Source: CAD feature listing. Evaluate the final solid. Frame: model axes, mm. A direction names the side the tool comes from. Round coordinates to 2 decimals unless told otherwise and drop trailing zeros. Write each loop counter-clockwise with the first axis right and the second up, starting at its lowest first coordinate (ties: lowest second). Pieces come first, ordered by that corner, then holes. Notation, with made-up numbers: M -5.5,-15.75 L -1.5,-15.75 A11 cw -1.5,-8.75 Z; hole C -19,-1.5 d9. An arc over 180 degrees is marked long. Answer in a Markdown table with one row per item. Add a question column.
Item 1: Contact query for flat-ended pins moving along their axis: pin 1 (0.5 mm diameter, centred on x = 37, y = 32.5, fed in from -Z); pin 2 (0.5 mm diameter, centred on x = 52.5, z = 2, fed in from +Y); pin 3 (2.5 mm diameter, centred on x = 48, y = 10, fed in from +Z); pin 4 (1.7 mm diameter, centred on x = 55, y = 30.5, fed in from -Z). Output: stop coordinate, or through.
Item 2: Cut plane A-A on x = 48. Return loops of the section in (y, z), and give its area (3 significant figures).
Item 3: Mould query, pull axis X, two halves, no side actions, for faces 6 (the face through (61.802, 0.713, 2.958)), 7 (the face through (0, 17, 4)), 8 (the face through (39, 17, 8)). Classes: released by +X, released by -X, zero draft, split by the parting line, or undercut.
Item 4: Cut plane D-D on x = 66.5. Return loops of the section in (y, z).
Item 5: Material intervals for probe 1 along X at (y, z) = (3, 2.25); probe 2 along Y at (x, z) = (73, 5.25); probe 3 along Y at (x, z) = (23, 7), sorted ascending.
Item 6: Cut plane C-C on x = 57. Return loops of the section in (y, z).
Item 7: Cut plane B-B on y = 25. Return loops of the section in (x, z).
Item 8: Set-up query: faces 1 (the face through (25, 6, 6)), 2 (the face through (52.35, 10.06, 2.22)), 3 (the face through (40, 33.2, 3)), 4 (the face through (76.74, 6.45, 3.94)), 5 (the face through (41, 33, 2.5)). Return all of +Z, -Z, +X, -X, +Y, -Y with unobstructed straight access to the full face (end or side cutting, diameter ignored); none if empty.
from build123d import *

# Parameters (mm, degrees)
SKETCH_2_W           = 80
SKETCH_2_H           = 34
SKETCH_2_R           = 4.05
EXTRUDE_1_DEPTH      = 8
SKETCH_3_R           = 2.55
CUT_EXTRUDE_1_DEPTH  = 88.292611371
CUT_EXTRUDE_2_DEPTH  = 88.292611371
SKETCH_5_R           = 1.55
CUT_EXTRUDE_3_DEPTH  = 88.292611371
CUT_EXTRUDE_4_DEPTH  = 6
CUT_EXTRUDE_5_DEPTH  = 4.5
SKETCH_20_R          = 5.5
CUT_EXTRUDE_12_DEPTH = 4.5
SKETCH_11_R          = 1.55
CUT_EXTRUDE_7_DEPTH  = 88.292611371
CUT_EXTRUDE_11_DEPTH = 2


with BuildPart() as part:
    # 草图2 → 凸台-拉伸1 (new body)
    with BuildSketch(Plane.XY):
        with Locations((40, 17)):
            Rectangle(SKETCH_2_W, SKETCH_2_H)
        with Locations((7, 8)):
            Circle(SKETCH_2_R, mode=Mode.SUBTRACT)
        with Locations((40, 10)):
            Circle(SKETCH_2_R, mode=Mode.SUBTRACT)
        with Locations((73, 8)):
            Circle(SKETCH_2_R, mode=Mode.SUBTRACT)
    extrude(amount=EXTRUDE_1_DEPTH)

    # 草图3 → 切除-拉伸1 (cut, through all)
    with BuildSketch(Plane.XY.offset(8)):
        with Locations((23, 8)):
            Circle(SKETCH_3_R)
        with Locations((57, 8)):
            Circle(SKETCH_3_R)
    extrude(amount=-CUT_EXTRUDE_1_DEPTH, mode=Mode.SUBTRACT)

    # 草图4 → 切除-拉伸2 (cut, through all)
    with BuildSketch(Plane(origin=(80, 0, 0), x_dir=(0, 0, -1), z_dir=(1, 0, 0))):
        Polygon((-1.5, 32.2), (-2.5, 32.2), (-2.5, 34), (0, 34), (0, 28.8), (-1.5, 28.8), align=None)
    extrude(amount=-CUT_EXTRUDE_2_DEPTH, mode=Mode.SUBTRACT)

    # 草图5 → 切除-拉伸3 (cut, through all)
    with BuildSketch(Plane.XY.offset(8)):
        with Locations((48, 10)):
            Circle(SKETCH_5_R)
        with Locations((32, 10)):
            Circle(SKETCH_5_R)
    extrude(amount=-CUT_EXTRUDE_3_DEPTH, mode=Mode.SUBTRACT)

    # 草图7 → 切除-拉伸4 (cut)
    with BuildSketch(Plane(origin=(0, 0, 0), x_dir=(-1, 0, 0), z_dir=(0, 0, -1))):
        with BuildLine():
            Line((-27.05, 10), (-27.05, 2.5))
            ThreePointArc((-27.05, 2.5), (-27.782233047, 0.732233047), (-29.55, 0))
            Line((-29.55, 0), (-16.45, 0))
            ThreePointArc((-16.45, 0), (-18.217766953, 0.732233047), (-18.95, 2.5))
            Line((-18.95, 2.5), (-18.95, 10))
            ThreePointArc((-18.95, 10), (-23, 14.05), (-27.05, 10))
        make_face()
        with BuildLine():
            Line((-61.05, 2.5), (-61.05, 10))
            ThreePointArc((-61.05, 10), (-57, 14.05), (-52.95, 10))
            Line((-52.95, 10), (-52.95, 2.5))
            ThreePointArc((-52.95, 2.5), (-52.217766953, 0.732233047), (-50.45, 0))
            Line((-50.45, 0), (-63.55, 0))
            ThreePointArc((-63.55, 0), (-61.782233047, 0.732233047), (-61.05, 2.5))
        make_face()
    extrude(amount=-CUT_EXTRUDE_4_DEPTH, mode=Mode.SUBTRACT)

    # 草图8 → 切除-拉伸5 (cut)
    with BuildSketch(Plane(origin=(0, 0, 0), x_dir=(-1, 0, 0), z_dir=(0, 0, -1))):
        with BuildLine():
            Line((-30.5, 12.85), (-49.5, 12.85))
            ThreePointArc((-49.5, 12.85), (-52.35, 10), (-49.5, 7.15))
            Line((-49.5, 7.15), (-30.5, 7.15))
            ThreePointArc((-30.5, 7.15), (-27.65, 10), (-30.5, 12.85))
        make_face()
    extrude(amount=-CUT_EXTRUDE_5_DEPTH, mode=Mode.SUBTRACT)

    # 草图20 → 切除-拉伸12 (cut)
    with BuildSketch(Plane(origin=(0, 0, 0), x_dir=(-1, 0, 0), z_dir=(0, 0, -1))):
        with Locations((-40, 10)):
            Circle(SKETCH_20_R)
    extrude(amount=-CUT_EXTRUDE_12_DEPTH, mode=Mode.SUBTRACT)

    # 草图11 → 切除-拉伸7 (cut, through all)
    with BuildSketch(Plane(origin=(0, 0, 0), x_dir=(-1, 0, 0), z_dir=(0, 0, -1))):
        with Locations((-60, 25)):
            Circle(SKETCH_11_R)
        with Locations((-20, 25)):
            Circle(SKETCH_11_R)
    extrude(amount=-CUT_EXTRUDE_7_DEPTH, mode=Mode.SUBTRACT)

    # 草图19 → 切除-拉伸11 (cut)
    with BuildSketch(Plane(origin=(0, 0, 2.5), x_dir=(-1, 0, 0), z_dir=(0, 0, -1))):
        with BuildLine():
            Line((-25, 34), (-55.247938178, 34))
            Line((-55.247938178, 34), (-55.247938178, 33.2))
            ThreePointArc((-55.247938178, 33.2), (-54.747938178, 32.7), (-54.247938178, 33.2))
            Line((-54.247938178, 33.2), (-26, 33.2))
            ThreePointArc((-26, 33.2), (-25.5, 32.7), (-25, 33.2))
            Line((-25, 33.2), (-25, 34))
        make_face()
    extrude(amount=-CUT_EXTRUDE_11_DEPTH, mode=Mode.SUBTRACT)


solid = part.part
Results below:
| question | item | result |
|---|---|---|
| 1 | pin 1 | z = 2.5 |
| 1 | pin 2 | y = 32.2 |
| 1 | pin 3 | through |
| 1 | pin 4 | z = 1.5 |
| 2 | outline | M 0,0 L 7.15,0 L 7.15,4.5 L 8.45,4.5 L 8.45,8 L 0,8 Z; M 11.55,4.5 L 12.85,4.5 L 12.85,0 L 28.8,0 L 28.8,1.5 L 32.2,1.5 L 32.2,2.5 L 33.2,2.5 L 33.2,4.5 L 34,4.5 L 34,8 L 11.55,8 Z |
| 2 | area | 224 mm2 |
| 3 | face 6 | undercut |
| 3 | face 7 | released by -X |
| 3 | face 8 | zero draft |
| 4 | outline | M 0,0 L 28.8,0 L 28.8,1.5 L 32.2,1.5 L 32.2,2.5 L 34,2.5 L 34,8 L 0,8 Z |
| 5 | probe 1 | 0 to 18.95, 27.05 to 52.95, 61.05 to 80 |
| 5 | probe 2 | 0 to 3.95, 12.05 to 34 |
| 5 | probe 3 | 0 to 5.45, 10.55 to 34 |
| 6 | outline | M 0,6 L 5.45,6 L 5.45,8 L 0,8 Z; M 10.55,6 L 14.05,6 L 14.05,0 L 28.8,0 L 28.8,1.5 L 32.2,1.5 L 32.2,2.5 L 34,2.5 L 34,8 L 10.55,8 Z |
| 7 | outline | M 0,0 L 18.45,0 L 18.45,8 L 0,8 Z; M 21.55,0 L 58.45,0 L 58.45,8 L 21.55,8 Z; M 61.55,0 L 80,0 L 80,8 L 61.55,8 Z |
| 8 | face 1 | -Z, -Y |
| 8 | face 2 | -Z |
| 8 | face 3 | -Z, +Y |
| 8 | face 4 | +Z, -Z |
| 8 | face 5 | -Z, +X, -X, +Y |
